from build123d import *

# Parameters (mm, degrees)
ESQUISSE1_W             = 42
ESQUISSE1_H             = 42
ESQUISSE1_R             = 11.5
ESQUISSE1_R_2           = 1.75
ESQUISSE1_W_2           = 7.5
ESQUISSE1_H_2           = 18
BOSS_EXTRU_1_DEPTH      = 9
ESQUISSE9_R             = 2.25
ENL_V_MAT_EXTRU_2_DEPTH = 17
ENL_V_MAT_EXTRU_3_DEPTH = 4.5
ESQUISSE11_R            = 3.75
ENL_V_MAT_EXTRU_4_DEPTH = 4.5
CONG_1_R                = 5
ESQUISSE12_R            = 1.75
ENL_V_MAT_EXTRU_5_DEPTH = 10
ENL_V_MAT_EXTRU_8_DEPTH = 4.5
ESQUISSE15_W            = 7
ESQUISSE15_H            = 5
ENL_V_MAT_EXTRU_9_DEPTH = 10
CONG_2_R                = 2.5


with BuildPart() as part:
    # Esquisse1 → Boss.-Extru.1 (new body)
    # profile 1 of 2: a face of its own
    with BuildSketch(Plane.XY):
        with Locations((-21, -21)):
            Rectangle(ESQUISSE1_W, ESQUISSE1_H)
        with Locations((-21, -21)):
            Circle(ESQUISSE1_R, mode=Mode.SUBTRACT)
        with Locations((-36.5, -36.5)):
            Circle(ESQUISSE1_R_2, mode=Mode.SUBTRACT)
        with Locations((-5.5, -36.5)):
            Circle(ESQUISSE1_R_2, mode=Mode.SUBTRACT)
        with Locations((-5.5, -5.5)):
            Circle(ESQUISSE1_R_2, mode=Mode.SUBTRACT)
        with Locations((-36.5, -5.611040912)):
            Circle(ESQUISSE1_R_2, mode=Mode.SUBTRACT)
    # profile 2 of 2: a face of its own
    with BuildSketch(Plane.XY):
        with Locations((-45.75, -21)):
            Rectangle(ESQUISSE1_W_2, ESQUISSE1_H_2)
    extrude(amount=BOSS_EXTRU_1_DEPTH)

    # Esquisse9 → Enlèv. mat.-Extru.2 (cut)
    with BuildSketch(Plane.XY.offset(9)):
        with Locations((-44.5, -21)):
            Circle(ESQUISSE9_R)
        with Locations((-37.5, -21)):
            Circle(ESQUISSE9_R)
    extrude(amount=-ENL_V_MAT_EXTRU_2_DEPTH, mode=Mode.SUBTRACT)

    # Esquisse10 → Enlèv. mat.-Extru.3 (cut)
    with BuildSketch(Plane(origin=(0, 0, 0), x_dir=(-1, 0, 0), z_dir=(0, 0, -1))):
        Polygon((44.5, -25.330127019), (48.25, -23.165063509), (48.25, -18.834936491), (44.5, -16.669872981), (40.75, -18.834936491), (40.75, -23.165063509), align=None)
        Polygon((37.5, -25.330127019), (41.25, -23.165063509), (41.25, -18.834936491), (37.5, -16.669872981), (33.75, -18.834936491), (33.75, -23.165063509), align=None)
    extrude(amount=-ENL_V_MAT_EXTRU_3_DEPTH, mode=Mode.SUBTRACT)

    # Esquisse11 → Enlèv. mat.-Extru.4 (cut)
    with BuildSketch(Plane.XY.offset(9)):
        with Locations((-36.5, -5.611040912)):
            Circle(ESQUISSE11_R)
        with Locations((-5.5, -5.5)):
            Circle(ESQUISSE11_R)
        with Locations((-5.5, -36.5)):
            Circle(ESQUISSE11_R)
        with Locations((-36.5, -36.5)):
            Circle(ESQUISSE11_R)
    extrude(amount=-ENL_V_MAT_EXTRU_4_DEPTH, mode=Mode.SUBTRACT)

    # Congé1
    cong_1_edges = [part.edges().sort_by_distance(p)[0] for p in [
        (0, 0, 4.5),
        (0, -42, 4.5),
        (-42, -42, 4.5),
        (-42, 0, 4.5),
    ]]
    fillet(cong_1_edges, radius=CONG_1_R)

    # Esquisse12 → Enlèv. mat.-Extru.5 (cut)
    with BuildSketch(Plane.XY.offset(9)):
        with Locations((-24, -38)):
            Circle(ESQUISSE12_R)
        with Locations((-18, -38)):
            Circle(ESQUISSE12_R)
        with Locations((-24, -4)):
            Circle(ESQUISSE12_R)
        with Locations((-18, -4)):
            Circle(ESQUISSE12_R)
    extrude(amount=-ENL_V_MAT_EXTRU_5_DEPTH, mode=Mode.SUBTRACT)

    # Esquisse14 → Enlèv. mat.-Extru.8 (cut)
    with BuildSketch(Plane(origin=(0, 0, 0), x_dir=(-1, 0, 0), z_dir=(0, 0, -1))):
        Polygon((27, -39.732050808), (27, -36.267949192), (24, -34.535898385), (21, -36.267949192), (18, -34.535898385), (15, -36.267949192), (15, -39.732050808), (18, -41.464101615), (21, -39.732050808), (24, -41.464101615), align=None)
        Polygon((27, -5.732050808), (27, -2.267949192), (24, -0.535898385), (21, -2.267949192), (18, -0.535898385), (15, -2.267949192), (15, -5.732050808), (18, -7.464101615), (21, -5.732050808), (24, -7.464101615), align=None)
    extrude(amount=-ENL_V_MAT_EXTRU_8_DEPTH, mode=Mode.SUBTRACT)

    # Esquisse15 → Enlèv. mat.-Extru.9 (cut)
    with BuildSketch(Plane(origin=(0, 0, 0), x_dir=(0, 0, -1), z_dir=(1, 0, 0))):
        with Locations((-5.5, -21)):
            Rectangle(ESQUISSE15_W, ESQUISSE15_H)
    extrude(amount=-ENL_V_MAT_EXTRU_9_DEPTH, mode=Mode.SUBTRACT)

    # Congé2
    cong_2_edges = [part.edges().sort_by_distance(p)[0] for p in [
        (-4.88751392, -23.5, 2),
        (-4.88751392, -18.5, 2),
    ]]
    fillet(cong_2_edges, radius=CONG_2_R - 0.0001)  # a hair under: the kernel refuses the full size


solid = part.part
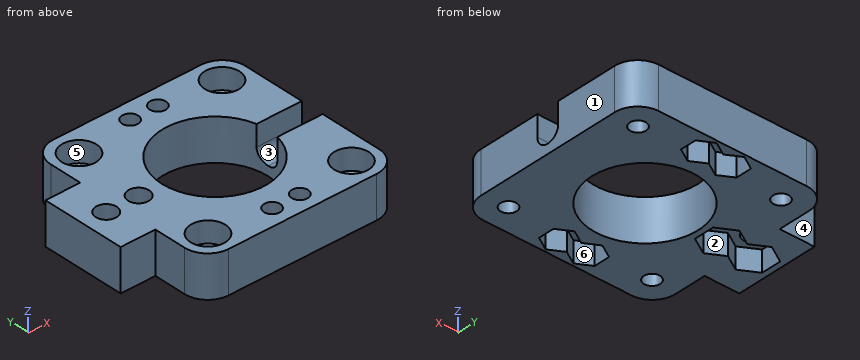
Here's how the part is built. I have some questions about the finished solid (model axes, mm). Face numbers are marked on the shaded views. A direction names the side the tool comes from. Round coordinates to 2 decimals unless told otherwise and drop trailing zeros. Write each loop counter-clockwise with the first axis right and the second up, starting at its lowest first coordinate (ties: lowest second). Pieces come first, ordered by that corner, then holes.
1. For the marked faces 4, 5 and 6, which set-ups out of +Z, -Z, +X, -X, +Y, -Y let a thin tool reach every point of the face, with its end or its side?
2. Suppose I cut it at D-D (y = -22.5). List the corners of the cut face in (x, z) for me.
3. I need wall thicknesses on L1, parallel to X at y = -36.5, z = 3.35; L2, parallel to X at y = -23, z = 1; L3, parallel to Y at x = -36, z = 0.75. Which ranges of each line are inside material? Lowest first, please.
4. Will these pins go through, and if not, where does the flat tip stop? pin 1 Ø4 at (y, z) = (-3.5, 3) entering from -X; pin 2 Ø4 at (x, z) = (-46, 5) entering from +Y; pin 3 Ø7 at (x, y) = (-5.5, -5.5) entering from +Z.
5. If we mould it in two halves opening along X, with no side actions, what happens to the marked faces 1, 2 and 3? For each: released by +X, released by -X, zero draft, split by the parting line, or undercut.
6. Suppose I cut it at A-A (x = -13). List the corners of the cut face in (y, z) for me, and give its area (3 significant figures).
7. Suppose I cut it at B-B (y = -28). List the corners of the cut face in (x, z) for me.
8. Suppose I cut it at C-C (z = 6.75). State how many separate pieces and enclosed holes the cut face has, and give its area (3 significant figures).
Answer sheet:
1. face 4: +Z, -Z, -X, +Y
1. face 5: +Z
1. face 6: -Z
2. outline: (-49.5, 0) - (-48.25, 0) - (-48.25, 4.5) - (-46.18, 4.5) - (-46.18, 9) - (-49.5, 9) - close; (-42.82, 4.5) - (-39.18, 4.5) - (-39.18, 9) - (-42.82, 9) - close; (-35.82, 4.5) - (-33.75, 4.5) - (-33.75, 0) - (-32.4, 0) - (-32.4, 9) - (-35.82, 9) - close; (-9.6, 0) - (0, 0) - (0, 2.5) - (-9.6, 2.5) - close
3. L1: x = -42 to -38.25, -34.75 to -27, -15 to -7.25, -3.75 to 0
3. L2: x = -49.5 to -48.25, -33.75 to -32.32, -9.68 to 0
3. L3: y = -42 to -38.18, -34.82 to -24.46, -17.54 to -7.29, -3.93 to 0
4. pin 1: stops at x = -42
4. pin 2: stops at y = -12
4. pin 3: stops at z = 4.5
5. face 1: released by +X
5. face 2: undercut
5. face 3: zero draft
6. outline: (-42, 0) - (-29.26, 0) - (-29.26, 9) - (-42, 9) - close; (-12.74, 0) - (0, 0) - (0, 9) - (-12.74, 9) - close
6. area: 229 mm2
7. outline: (-49.5, 0) - (-30.12, 0) - (-30.12, 9) - (-49.5, 9) - close; (-11.88, 0) - (0, 0) - (0, 9) - (-11.88, 9) - close
8. separate pieces: 1
8. enclosed holes: 10
8. area: 1,170 mm2
